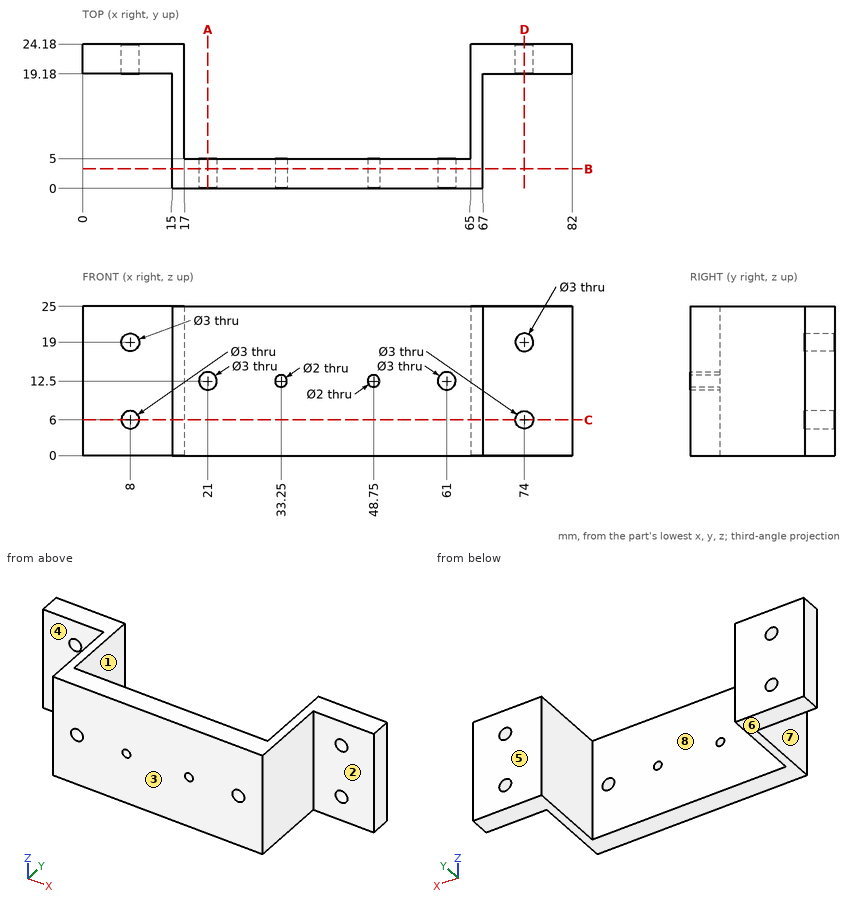
Drawing for the job (mm, zero at the part's lowest x, y, z). A direction names the side the tool comes from. Coordinates: 2 decimals unless noted, no trailing zeros. Write each loop counter-clockwise with the first axis right and the second up, starting at its lowest first coordinate (ties: lowest second). Pieces come first, ordered by that corner, then holes. Notation, with made-up numbers: (40, -23) - (46, -23) arc R26 cw to (46, 5) - close; hole circle Ø5 at (26.25, 32). An arc over 180 degrees is marked (long way). Write each question's results on one line, items separated by ' | '. Start each with the question number.
1) Flat gauge pins, fed straight in: P1, Ø6, axis at y = 5.5, z = 7, coming from the -X side; P2, Ø5, axis at x = 26.5, z = 22.5, coming from the +Y side; P3, Ø7.5, axis at x = 11, z = 7, coming from the -Y side. Where does each tip first touch, or does it go through?
2) Cut at D-D (x = 74). Write the cut outline in (y, z).
3) Cut at B-B (y = 3.25). Write the cut outline in (x, z).
4) Cut at A-A (x = 21). Write the cut outline in (y, z).
5) Mould opens along X. For the marked faces 6, 7 and 8 say: pulls with the +X half, pulls with the -X half, needs draft (parallel to the pull), parting line crosses it, or undercut.
6) 3-axis set-ups, long thin cutter, end or side, ignore diameter. For the marked faces 1, 2, 3, 4 and 5: which of +Z, -Z, +X, -X, +Y, -Y reach the whole face in a straight line?
7) Probe line 1 along Z through (x, y) = (74, 23); line 2 along X through (y, z) = (2.6, 12.5); line 3 along X through (y, z) = (20.8, 19). List the from-to ranges inside material, lowest first. Write a range as from..to.
8) Cut at C-C (z = 6). Write the cut outline in (x, y).
Returned:
1) P1: x = 15 | P2: y = 5 | P3: y = 19.18
2) outline: (19.18, 0) - (24.18, 0) - (24.18, 4.5) - (19.18, 4.5) - close; (19.18, 7.5) - (24.18, 7.5) - (24.18, 17.5) - (19.18, 17.5) - close; (19.18, 20.5) - (24.18, 20.5) - (24.18, 25) - (19.18, 25) - close
3) outline: (15, 0) - (67, 0) - (67, 25) - (15, 25) - close; hole circle Ø3 at (21, 12.5); hole circle Ø2 at (33.25, 12.5); hole circle Ø2 at (48.75, 12.5); hole circle Ø3 at (61, 12.5)
4) outline: (0, 0) - (5, 0) - (5, 11) - (0, 11) - close; (0, 14) - (5, 14) - (5, 25) - (0, 25) - close
5) face 6: needs draft | face 7: pulls with the -X half | face 8: undercut
6) face 1: +Z, -Z, +Y | face 2: +Z, -Z, +X, -Y | face 3: +Z, -Z, +X, -X, -Y | face 4: +Z, -Z, -X, -Y | face 5: +Z, -Z, +X, -X, +Y
7) line 1: 0..4.5, 7.5..17.5, 20.5..25 | line 2: 15..19.5, 22.5..32.25, 34.25..47.75, 49.75..59.5, 62.5..67 | line 3: 0..6.5, 9.5..17, 65..72.5, 75.5..82
8) outline: (0, 19.18) - (6.5, 19.18) - (6.5, 24.18) - (0, 24.18) - close; (9.5, 19.18) - (15, 19.18) - (15, 0) - (67, 0) - (67, 19.18) - (72.5, 19.18) - (72.5, 24.18) - (65, 24.18) - (65, 5) - (17, 5) - (17, 24.18) - (9.5, 24.18) - close; (75.5, 19.18) - (82, 19.18) - (82, 24.18) - (75.5, 24.18) - close
